Could you check a few things on this model? Use its own coordinates, in mm. A direction names the side the tool comes from. Round coordinates to 2 decimals unless told otherwise and drop trailing zeros. Loops run counter-clockwise (first coordinate to the right, second up) from the corner with the lowest first, then second, coordinate; pieces in that order, holes last. Notation, with made-up numbers: (-4.75, 5.5) -> (53.25, 5.5) arc R12 ccw to (53.25, 9.5) -> close; hole circle Ø9 at (60, 46). An arc over 180 degrees is marked (long way). One line per item, written item: value.
from build123d import *

# Parameters (mm, degrees)
SKETCH1_R           = 8
BOSS_EXTRUDE1_DEPTH = 8
FILLET1_R           = 4
FILLET2_R           = 10
SKETCH2_R           = 2.1
CUT_EXTRUDE1_DEPTH  = 9


with BuildPart() as part:
    # Sketch1 → Boss-Extrude1 (new body)
    with BuildSketch(Plane(origin=(0, 0, 0), x_dir=(1, 0, 0), z_dir=(0, 1, 0))):
        with BuildLine():
            Line((-33, 0), (-44, 0))
            Line((-44, 0), (-42, -10))
            Line((-42, -10), (-24, -22.649503306))
            ThreePointArc((-24, -22.649503306), (30.66757245, 12.186057607), (-33, 0))
        make_face()
        with Locations((-1.62, -0.35)):
            Circle(SKETCH1_R, mode=Mode.SUBTRACT)
    extrude(amount=BOSS_EXTRUDE1_DEPTH)

    # Fillet1
    fillet1_edges = [part.edges().sort_by_distance(p)[0] for p in [
        (-33, 4, 0),
    ]]
    fillet(fillet1_edges, radius=FILLET1_R)

    # Fillet2
    fillet2_edges = [part.edges().sort_by_distance(p)[0] for p in [
        (-24, 4, 22.649503306),
        (-42, 4, 10),
    ]]
    fillet(fillet2_edges, radius=FILLET2_R)

    # Sketch2 → Cut-Extrude1 (cut, through all)
    with BuildSketch(Plane(origin=(0, 8, 0), x_dir=(1, 0, 0), z_dir=(0, 1, 0))):
        with Locations((-1.452372624, 13.648996431)):
            Circle(SKETCH2_R)
        with Locations((10.650920222, 6.644137969)):
            Circle(SKETCH2_R)
        with Locations((10.636181267, -7.340050335)):
            Circle(SKETCH2_R)
        with Locations((-1.481850533, -14.319380179)):
            Circle(SKETCH2_R)
        with Locations((-13.585143379, -7.314521718)):
            Circle(SKETCH2_R)
        with Locations((-13.570404425, 6.669666587)):
            Circle(SKETCH2_R)
    extrude(amount=-CUT_EXTRUDE1_DEPTH, mode=Mode.SUBTRACT)


solid = part.part
(1) If we section it at D-D, the plane z = -27: Please give me the cut outline in (x, y).
Recorded:
outline: (-18.97, 0) -> (18.97, 0) -> (18.97, 8) -> (-18.97, 8) -> close
(2) If we section it at A-A, the plane x = -1.62: Please give me the cut outline in (y, z), then the cut area to 3 significant figures.
Recorded:
outline: (0, -32.96) -> (8, -32.96) -> (8, -15.74) -> (0, -15.74) -> close; (0, -11.56) -> (8, -11.56) -> (8, -7.65) -> (0, -7.65) -> close; (0, 8.35) -> (8, 8.35) -> (8, 12.22) -> (0, 12.22) -> close; (0, 16.41) -> (8, 16.41) -> (8, 32.96) -> (0, 32.96) -> close
area: 332 mm²
(3) If I drill on L1, parallel to Z at x = 0, y = 4.5; L2, parallel to Z at x = -2, y = 4.75; L3, parallel to Z at x = 9, y = 4.75, over which ranges is the centre line in solid material (lowest first)?
Recorded:
L1: -33 to -15.17, -12.13 to -7.48, 8.18 to 12.83, 15.81 to 33
L2: -32.94 to -15.68, -11.62 to -7.64, 8.34 to 12.28, 16.35 to 32.94
L3: -31.75 to -7.94, -5.35 to 6.02, 8.66 to 31.75
(4) For faces 1 (the face through (-40, 4, 0)), 2 (the face through (-41.384, 4.056, 9.535)), which set-ups out of +Z, -Z, +X, -X, +Y, -Y let a thin tool reach every point of the face, with its end or its side?
Recorded:
face 1: -Z, -X, +Y, -Y
face 2: +Z, -X, +Y, -Y
(5) I'm going to push flat-ended pins straight in: pin 1 Ø4 at (x, y) = (-7, 7) entering from -Z; pin 2 Ø2 at (x, y) = (-42, 3) entering from -Z; pin 3 Ø2.5 at (x, z) = (-13.59, 7.31) entering from -Y; pin 4 Ø1 at (y, z) = (2.5, -18) entering from +X. Where does each tip first touch, or does it pass through?
Recorded:
pin 1: z = -32.62
pin 2: z = 0
pin 3: through
pin 4: x = 27.98
(6) If we section it at B-B, the plane x = 10.5: Please give me the cut outline in (y, z), then the cut area to 3 significant figures.
Recorded:
outline: (0, -31.28) -> (8, -31.28) -> (8, -8.74) -> (0, -8.74) -> close; (0, -4.55) -> (8, -4.55) -> (8, 5.24) -> (0, 5.24) -> close; (0, 9.44) -> (8, 9.44) -> (8, 31.28) -> (0, 31.28) -> close
area: 434 mm²
(7) Thinking about a two-plate mould opening in Z: for faces 3 (the face through (-31.848, 3.944, 17.134)), 4 (the face through (6.01, 3.94, -2.05)), 5 (the face through (-0.51, 4.06, 16.18)), 6 (the face through (3, 0, -8)), which applies, released by +Z, released by -Z, zero draft, split by the parting line, or undercut?
Recorded:
face 3: released by +Z
face 4: undercut
face 5: undercut
face 6: zero draft
(8) If we section it at C-C, the plane y = 7: Please give me the cut outline in (x, z), then the cut area to 3 significant figures.
Recorded:
outline: (-44, 0) -> (-36.78, 0) arc R4 cw to (-32.81, -3.57) arc R33 ccw (long way) to (-23.42, 23.24) arc R10 cw to (-24.77, 22.11) -> (-38.73, 12.3) arc R10 ccw to (-42.78, 6.08) -> close; hole circle Ø4.2 at (-13.59, 7.31); hole circle Ø4.2 at (-13.57, -6.67); hole circle Ø16 at (-1.62, 0.35); hole circle Ø4.2 at (-1.48, 14.32); hole circle Ø4.2 at (-1.45, -13.65); hole circle Ø4.2 at (10.64, 7.34); hole circle Ø4.2 at (10.65, -6.64)
area: 3,300 mm²
